For this review, take the finished solid that the model builds, in its own axes (mm). Coordinates: 2 decimals unless noted, no trailing zeros. Loops run counter-clockwise (first coordinate to the right, second up) from the corner with the lowest first, then second, coordinate; pieces in that order, holes last. Notation, with made-up numbers: M -2,-16.5 L 37,-16.5 A21 ccw 37,19.5 Z; hole C 83,51.5 d7. An arc over 180 degrees is marked long. Use one line per item in the form item = value.
```python
from build123d import *

# Parameters (mm, degrees)
F0_R     = 11.495248
F0_R_2   = 11
F1_DEPTH = 3


with BuildPart() as f1:
    # F0 (on Top) → F1 (new body)
    with BuildSketch(Plane.XY):
        with BuildLine():
            Line((34.073839, 28.946415), (28.237904, 32.489196))
            ThreePointArc((28.237904, 32.489196), (3.787903, 39.731164), (-21.466842, 36.203202))
            ThreePointArc((-21.466842, 36.203202), (-16.224646, 20.401304), (-20.807121, 4.395633))
            ThreePointArc((-20.807121, 4.395633), (-34.826813, 2.968602), (-42.10525, 15.035603))
            Line((-42.10525, 15.035603), (-42.255421, 8.210144))
            ThreePointArc((-42.255421, 8.210144), (-36.302149, -16.585162), (-20.619472, -36.692431))
            ThreePointArc((-20.619472, -36.692431), (-9.555725, -24.251607), (6.596831, -20.217312))
            ThreePointArc((6.596831, -20.217312), (14.842522, -31.645205), (8.031411, -43.982018))
            Line((8.031411, -43.982018), (14.017518, -40.69934))
            ThreePointArc((14.017518, -40.69934), (32.514246, -23.146002), (42.086313, 0.48923))
            ThreePointArc((42.086313, 0.48923), (25.78037, 3.850303), (14.21029, 15.821679))
            ThreePointArc((14.21029, 15.821679), (19.984291, 28.676604), (34.073839, 28.946415))
        make_face()
        with Locations((-21.527926, -11.295904)):
            Circle(F0_R, mode=Mode.SUBTRACT)
        with Locations((22.755247, -13.960625)):
            Circle(F0_R_2, mode=Mode.SUBTRACT)
        with BuildLine():
            ThreePointArc((-9.526279, 5.5), (0, 11), (9.526279, 5.5))
            ThreePointArc((9.526279, 5.5), (9.526279, -5.5), (0, -11))
            ThreePointArc((0, -11), (-9.526279, -5.5), (-9.526279, 5.5))
        make_face(mode=Mode.SUBTRACT)
        with Locations((0, 25.195053)):
            Circle(F0_R_2, mode=Mode.SUBTRACT)
    extrude(amount=F1_DEPTH)


solid = f1.part
```
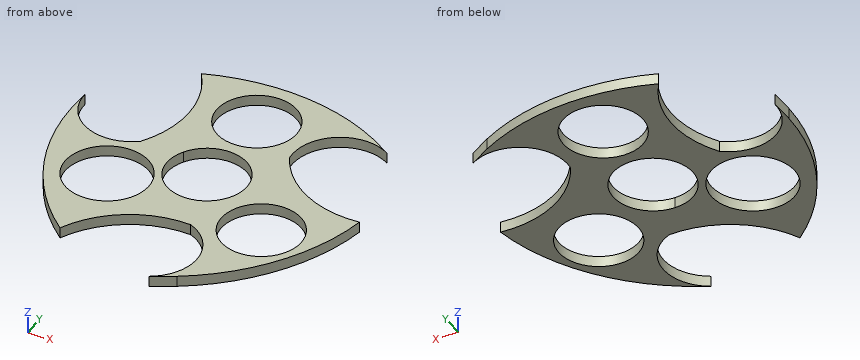
1. Consider section C-C on z = 2.2. Write out the cut boundary in (x, y).
Computed values:
outline = M -42.26,8.21 A60.21 ccw -20.62,-36.69 A28.21 cw 6.6,-20.22 A13.17 cw 8.03,-43.98 L 14.02,-40.7 A60.21 ccw 42.09,0.49 A28.21 cw 14.21,15.82 A13.17 cw 34.07,28.95 L 28.24,32.49 A60.21 ccw -21.47,36.2 A28.21 cw -20.81,4.4 A13.17 cw -42.11,15.04 Z; hole C -21.53,-11.3 d22.99; hole C 0,0 d22; hole C 0,25.2 d22; hole C 22.76,-13.96 d22
2. Consider section B-B on y = -6.5. Write out the cut boundary in (x, z), plus the area to 3 significant figures.
Computed values:
outline = M -40.09,0 L -31.97,0 L -31.97,3 L -40.09,3 Z; M -11.08,0 L -8.87,0 L -8.87,3 L -11.08,3 Z; M 8.87,0 L 14.67,0 L 14.67,3 L 8.87,3 Z; M 30.84,0 L 40.44,0 L 40.44,3 L 30.84,3 Z
area = 77.2 mm2
3. Wall thickness on line 1 along Y through (x, z) = (24, 1.85); line 2 along Y through (x, z) = (-8.5, 1.45); line 3 along X through (y, z) = (8, 1.2): over which ranges is each line inside the solid? List them lowest first. Write a range as from..to.
Computed values:
line_1 = -33.11..-24.89, -3.03..4.92, 30.45..34.6
line_2 = -23.64..-6.98, 6.98..18.21, 32.18..39.39
line_3 = -42.25..-40.25, -18.81..-7.55, 7.55..20.07
4. Consider section A-A on x = 26.5. Write out the cut boundary in (y, z).
Computed values:
outline = M -30.62,0 L -24.3,0 L -24.3,3 L -30.62,3 Z; M -3.62,0 L 3.47,0 L 3.47,3 L -3.62,3 Z; M 30.84,0 L 33.41,0 L 33.41,3 L 30.84,3 Z
5. For pin 1 Ø2 at (x, y) = (2, -21.5) entering from +Z, flat-tipped, find the tip position at first contact; note if it passes through.
Computed values:
pin_1 = through
6. Consider section D-D on y = 19. Write out the cut boundary in (x, z).
Computed values:
outline = M -16.23,0 L -9.09,0 L -9.09,3 L -16.23,3 Z; M 9.09,0 L 14.14,0 L 14.14,3 L 9.09,3 Z
